Autodesk Inventor part; units mm, degrees
ref_plane "YZ Plane" through (0, 0, 0) normal (1, 0, 0) x (0, 1, 0)
ref_plane "XZ Plane" through (0, 0, 0) normal (0, 1, 0) x (-1, 0, 0)
ref_plane "XY Plane" through (0, 0, 0) normal (0, 0, 1) x (1, 0, 0)
sketch "Sketch1" plane through (0, 0, 0) normal (0, 1, 0) x (-1, 0, 0)
  line L0 (-38.1051, 6) -> (13.8564, 36)
  line L1 (-38.1051, -6) -> (13.8564, -36)
  line L2 (24.2487, 30) -> (24.2487, -30)
  line L3 (24.2487, 30) -> (13.8564, 36)
  line L4 (24.2487, -30) -> (13.8564, -36)
  line L5 (-38.1051, 6) -> (-38.1051, -6)
  line L6 (19.0526, 6) -> (19.0526, -6)
  line L7 (21.0526, -6) -> (21.0526, 6)
  arc A0 (21.0526, 6) -> (19.0526, 6) centre (20.0526, 6) ccw
  arc A1 (19.0526, -6) -> (21.0526, -6) centre (20.0526, -6) ccw
  line L8 (-2.5, 12.5) -> (-2.5, -11.5)
  line L9 (-1.5, -12.5) -> (1.5, -12.5)
  line L10 (2.5, -11.5) -> (2.5, 12.5)
  line L11 (-4, 12.5) -> (-4, -12.5)
  line L12 (-2.5, -14) -> (2.5, -14)
  line L13 (4, -12.5) -> (4, 12.5)
  arc A2 (4, 12.5) -> (2.5, 12.5) centre (3.25, 12.5) ccw
  arc A3 (-2.5, 12.5) -> (-4, 12.5) centre (-3.25, 12.5) ccw
  arc A4 (2.5, -14) -> (4, -12.5) centre (2.5, -12.5) ccw
  arc A5 (-4, -12.5) -> (-2.5, -14) centre (-2.5, -12.5) ccw
  arc A6 (-2.5, -11.5) -> (-1.5, -12.5) centre (-1.5, -11.5) ccw
  arc A7 (1.5, -12.5) -> (2.5, -11.5) centre (1.5, -11.5) ccw
  point P0 (0, 0)
  point P1 (0, 0)
extrude "Extrusion1" add sketch "Sketch1" along normal blind 1.6
properties part number "PCB_Bottom"
Can you work these out from the model? Positions are in its coordinate system, mm. A direction names the side the tool comes from. Coordinates: 2 decimals unless noted, no trailing zeros. Loops run counter-clockwise (first coordinate to the right, second up) from the corner with the lowest first, then second, coordinate; pieces in that order, holes last. Notation, with made-up numbers: M 40,-19.75 L 78,-19.75 A25 cw 78,-3.75 Z; hole C 2.5,44.5 d1. An arc over 180 degrees is marked long. Answer as CSV lines item,"result". Start each with the question number.
1. Suppose I cut it at D-D, the plane z = 24.5. List the corners of the cut face in (x, y) for me, plus the area to 3 significant figures.
2. Thinking about a two-plate mould opening in X: for faces 1 (the face through (-24.249, 1, 0)), 2 (the face through (0, 0, 1)), 3 (the face through (0, 1, -12.5)), 4 (the face through (-19.053, 1, 0)), which applies, +X half, -X half, draft (parallel to the pull), parting line (faces both ways), or undercut?
3. Suppose I cut it at B-B, the plane y = 1.2. List the corners of the cut face in (x, z) for me, plus the area to 3 significant figures.
4. Suppose I cut it at C-C, the plane x = 31.5. List the corners of the cut face in (y, z) for me, plus the area to 3 significant figures.
5. For faces 5 (the face through (-21.053, 1, 0)), 6 (the face through (12.49, 0.79, 20.79)), which set-ups out of +Z, -Z, +X, -X, +Y, -Y let a thin tool reach every point of the face, with its end or its side?
6. Suppose I cut it at A-A, the plane z = 5. List the corners of the cut face in (x, y) for me.
7. For pin 1 Ø0.5 at (x, y) = (-1, 0.5) entering from +Z; pin 2 Ø0.5 at (x, y) = (0.5, 0.5) entering from -Z, each with a flat end and sliding along its axis, tell me the tip position at first contact or that it passes through.
8. If I drill on probe 1 along X at (y, z) = (1.2, 4); probe 2 along X at (y, z) = (1.3, 8); probe 3 along X at (y, z) = (0.75, 10.5), over which ranges is the centre line in solid material (lowest first)? Write a range as [from, to].
Output:
1,outline,"M -24.25,0 L 6.06,0 L 6.06,1.6 L -24.25,1.6 Z"
1,area,"48.5 mm^2"
2,face 1,"-X half"
2,face 2,"draft"
2,face 3,"undercut"
2,face 4,"undercut"
3,outline,"M -24.25,-30 L -13.86,-36 L 38.11,-6 L 38.11,6 L -13.86,36 L -24.25,30 Z; hole M -21.05,-6 A1 ccw -19.05,-6 L -19.05,6 A1 ccw -21.05,6 Z; hole M -4,-12.5 A1.5 ccw -2.5,-14 L 2.5,-14 A1.5 ccw 4,-12.5 L 4,12.5 A0.75 ccw 2.5,12.5 L 2.5,-11.5 A1 cw 1.5,-12.5 L -1.5,-12.5 A1 cw -2.5,-11.5 L -2.5,12.5 A0.75 ccw -4,12.5 Z"
3,area,"2,750 mm^2"
4,outline,"M 0,-9.81 L 1.6,-9.81 L 1.6,9.81 L 0,9.81 Z"
4,area,"31.4 mm^2"
5,face 5,"+Y, -Y"
5,face 6,"+Z, +X, +Y, -Y"
6,outline,"M -24.25,0 L -21.05,0 L -21.05,1.6 L -24.25,1.6 Z; M -19.05,0 L -4,0 L -4,1.6 L -19.05,1.6 Z; M -2.5,0 L 2.5,0 L 2.5,1.6 L -2.5,1.6 Z; M 4,0 L 38.11,0 L 38.11,1.6 L 4,1.6 Z"
7,pin 1,"stops at z = 28.72"
7,pin 2,"stops at z = -27.86"
8,probe 1,"x = [-24.25, -21.05], [-19.05, -4], [-2.5, 2.5], [4, 38.11]"
8,probe 2,"x = [-24.25, -4], [-2.5, 2.5], [4, 34.64]"
8,probe 3,"x = [-24.25, -4], [-2.5, 2.5], [4, 30.31]"
